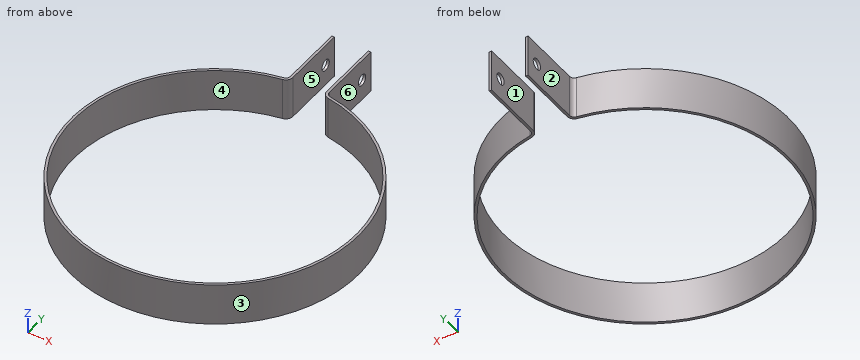
Autodesk Inventor part; units mm, degrees
ref_plane "YZ Plane" through (0, 0, 0) normal (1, 0, 0) x (0, 1, 0)
ref_plane "XZ Plane" through (0, 0, 0) normal (0, 1, 0) x (-1, 0, 0)
ref_plane "XY Plane" through (0, 0, 0) normal (0, 0, 1) x (1, 0, 0)
sketch "Sketch1" plane through (0, 0, 0) normal (0, 0, 1) x (1, 0, 0)
  line L0 (0, 0) -> (0, 19.8871) construction
  arc A0 (-8.0952, 49.3403) -> (8.0952, 49.3403) centre (0, 0) ccw
  arc A1 (-8.241, 50.2284) -> (8.241, 50.2284) centre (0, 0) ccw
  line L1 (-6, 74.4853) -> (-6, 51.8073)
  arc A2 (-8.0952, 49.3403) -> (-6, 51.8073) centre (-8.5, 51.8073) ccw
  arc A3 (-8.241, 50.2284) -> (-6.9, 51.8073) centre (-8.5, 51.8073) ccw
  line L2 (-6.9, 51.8073) -> (-6.9, 74.4853)
  line L3 (-6.9, 74.4853) -> (-6, 74.4853)
  line L4 (6, 74.4853) -> (6, 51.8073)
  arc A4 (6, 51.8073) -> (8.0952, 49.3403) centre (8.5, 51.8073) ccw
  arc A5 (6.9, 51.8073) -> (8.241, 50.2284) centre (8.5, 51.8073) ccw
  line L5 (6.9, 51.8073) -> (6.9, 74.4853)
  line L6 (6.9, 74.4853) -> (6, 74.4853)
  point P0 (-6.455, 50.3692)
  point P1 (6.455, 50.3692)
  dimension "d32" = 5
  dimension "d33" = 6
  dimension "d34" = 0.9
  dimension "d44" = 50
  dimension "d45" = 50.9
  dimension "d46" = 22.678
extrude "Extrusion1" add sketch "Sketch1" against normal blind 15
sketch "Sketch2" plane through (-6.9, 51.8073, 0) normal (-1, 0, 0) x (0, 0, 1)
  line L0 (0, 22.678) -> (-15, 22.678)
  line L1 (0, 22.678) -> (0, 0)
  point P0 (0, -51.8073)
  point P1 (-7.5, 17.878)
  dimension "d35" = 4.8
  dimension "d43" = 7.5
hole "Hole1" at (-6.9, 69.6853, -7.5) direction (1, 0, 0) diameter 4 depth 25 tip angle 137
properties part number "Banda de montaje"
Can you work these out from the model? Positions are in its coordinate system, mm. Face numbers are marked on the shaded views. A direction names the side the tool comes from. Coordinates: 2 decimals unless noted, no trailing zeros. Loops run counter-clockwise (first coordinate to the right, second up) from the corner with the lowest first, then second, coordinate; pieces in that order, holes last. Notation, with made-up numbers: (19.25, -21) - (78.25, -21) arc R26 cw to (78.25, 18) - close; hole circle Ø7 at (51.25, -1). An arc over 180 degrees is marked (long way). Answer as CSV lines item,"result". Start each with the question number.
1) For pin 1 (1 mm diameter, centred on x = 0, z = -4, fed in from +Y); pin 2 (8 mm diameter, centred on y = -21, z = -5.5, fed in from -X); pin 3 (1 mm diameter, centred on y = 26.5, z = -2, fed in from +X), each with a flat end and sliding along its axis, tell me the tip position at first contact or that it passes through.
2) Which directions (+Z, -Z, +X, -X, +Y, -Y) give clear straight access to the entire face, cutting with the end or side of a thin tool? Please do the marked faces 4, 5 and 6.
3) Suppose I cut it at C-C (x = 38). Please give me the cut outline in (y, z), plus the area to 3 significant figures.
4) Suppose I cut it at B-B (z = -7.5). Please give me the cut outline in (x, y), plus the area to 3 significant figures.
5) Suppose I cut it at D-D (z = -13.5). Please give me the cut outline in (x, y), plus the area to 3 significant figures.
6) Suppose I cut it at A-A (y = 0). Please give me the cut outline in (x, z), plus the area to 3 significant figures.
7) I need wall thicknesses on line 1 (X direction, y = 63.5, z = -2.25); line 2 (Y direction, x = -6.2, z = -7.5); line 3 (X direction, y = 30.5, z = -0.75). Which ranges of each line are inside material? Lowest first, please. Write a range as from..to.
8) Thinking about a two-plate mould opening in X: for the marked faces 1, 2 and 3, which applies, pulls with the +X half, pulls with the -X half, needs draft (parallel to the pull), parting line crosses it, or undercut?
Check result:
1,pin 1,"stops at y = -50"
1,pin 2,"stops at x = -47.98"
1,pin 3,"stops at x = 43.76"
2,face 4,"+Z, -Z"
2,face 5,"+Z, -Z, +Y"
2,face 6,"+Z, -Z, +X, +Y"
3,outline,"(-33.86, -15) - (-32.5, -15) - (-32.5, 0) - (-33.86, 0) - close; (32.5, -15) - (33.86, -15) - (33.86, 0) - (32.5, 0) - close"
3,area,"41.1 mm²"
4,outline,"(-8.24, 50.23) arc R50.9 ccw (long way) to (8.24, 50.23) arc R1.6 cw to (6.9, 51.81) - (6.9, 67.69) - (6, 67.69) - (6, 51.81) arc R2.5 ccw to (8.1, 49.34) arc R50 cw (long way) to (-8.1, 49.34) arc R2.5 ccw to (-6, 51.81) - (-6, 67.69) - (-6.9, 67.69) - (-6.9, 51.81) arc R1.6 cw to start; (-6.9, 71.69) - (-6, 71.69) - (-6, 74.49) - (-6.9, 74.49) - close; (6, 71.69) - (6.9, 71.69) - (6.9, 74.49) - (6, 74.49) - close"
4,area,"309 mm²"
5,outline,"(-8.24, 50.23) arc R50.9 ccw (long way) to (8.24, 50.23) arc R1.6 cw to (6.9, 51.81) - (6.9, 74.49) - (6, 74.49) - (6, 51.81) arc R2.5 ccw to (8.1, 49.34) arc R50 cw (long way) to (-8.1, 49.34) arc R2.5 ccw to (-6, 51.81) - (-6, 74.49) - (-6.9, 74.49) - (-6.9, 51.81) arc R1.6 cw to start"
5,area,"317 mm²"
6,outline,"(-50.9, -15) - (-50, -15) - (-50, 0) - (-50.9, 0) - close; (50, -15) - (50.9, -15) - (50.9, 0) - (50, 0) - close"
6,area,"27.0 mm²"
7,line 1,"x = -6.9..-6, 6..6.9"
7,line 2,"y = -50.52..-49.61, 50.83..67.69, 71.69..74.49"
7,line 3,"x = -40.75..-39.62, 39.62..40.75"
8,face 1,"undercut"
8,face 2,"pulls with the -X half"
8,face 3,"parting line crosses it"
